```python
from build123d import *

# Parameters (mm, degrees)
BOSS_EXTRUDE1_DEPTH = 2
SKETCH2_R           = 10
CUT_EXTRUDE1_DEPTH  = 434.878349498
SKETCH4_OUTSIDE_W   = 492.732
SKETCH4_OUTSIDE_H   = 440.742
CUT_EXTRUDE2_DEPTH  = 3


with BuildPart() as part:
    # Sketch1 → Boss-Extrude1 (new body)
    with BuildSketch(Plane(origin=(0, 0, 0), x_dir=(1, 0, 0), z_dir=(0, 1, 0))):
        Polygon((-132.853430349, -388.070415552), (132.853430349, -388.070415552), (194.030344885, -282.108891325), (61.176914536, -52), (-61.176914536, -52), (-194.030344885, -282.108891325), align=None)
    extrude(amount=BOSS_EXTRUDE1_DEPTH)

    # Sketch2 → Cut-Extrude1 (cut, through all)
    with BuildSketch(Plane(origin=(0, 2, 0), x_dir=(1, 0, 0), z_dir=(0, 1, 0))):
        with Locations(Location((0, -240.726435625, 0), (0, 0, 270))):
            Circle(SKETCH2_R)
    extrude(amount=-CUT_EXTRUDE1_DEPTH, mode=Mode.SUBTRACT)

    # Sketch4 outside → Cut-Extrude2 (cut)
    with BuildSketch(Plane(origin=(0, 2, 0), x_dir=(1, 0, 0), z_dir=(0, 1, 0))):
        with Locations((0, -220.035)):
            Rectangle(SKETCH4_OUTSIDE_W, SKETCH4_OUTSIDE_H)
        Polygon((-75.405516164, -76.644660941), (-40.050177105, -112), (40.050177105, -112), (75.405516164, -76.644660941), (179.801743257, -257.464230384), (131.505451943, -270.405182639), (91.455274838, -339.774124237), (104.396227093, -388.070415552), (-104.396227093, -388.070415552), (-91.455274838, -339.774124237), (-131.505451943, -270.405182639), (-179.801743257, -257.464230384), align=None, mode=Mode.SUBTRACT)
    extrude(amount=-CUT_EXTRUDE2_DEPTH, mode=Mode.SUBTRACT)


solid = part.part
```
Source: CAD feature listing. Evaluate the final solid. Frame: model axes, mm. A direction names the side the tool comes from. Round coordinates to 2 decimals unless told otherwise and drop trailing zeros. Loops run counter-clockwise (first coordinate to the right, second up) from the corner with the lowest first, then second, coordinate; pieces in that order, holes last. Notation, with made-up numbers: M 6,-10.75 L 17,-10.75 A18 ccw 17,-5.75 Z; hole C 62,52.25 d7. An arc over 180 degrees is marked long. Use a Markdown table: item, result. Add a question column.
1. Set-up query: faces 4 (the flat face through (-98.016, 1.014, 364.26)), 5 (the flat face through (-57.98, 1.01, 94.07)), 6 (the flat face through (111.761, 1.014, 304.604)). Return all of +Z, -Z, +X, -X, +Y, -Y with unobstructed straight access to the full face (end or side cutting, diameter ignored); none if empty.
2. Cut plane D-D, the plane x = 64. Output: boundary loops of the cut face in (y, z), and give its area (3 significant figures).
3. Cut plane A-A, the plane x = 0. Output: boundary loops of the cut face in (y, z).
4. Cut plane B-B, the plane y = 1.05. Output: boundary loops of the cut face in (x, z).
5. Ray query, line 1 along Z through (x, y) = (-74, 0.2); line 2 along X through (y, z) = (1.15, 91); line 3 along X through (y, z) = (0.8, 245.5). Return the intervals inside material, ascending. Write a range as [from, to].
6. Cut plane C-C, the plane z = 295.5. Output: boundary loops of the cut face in (x, y), and give its area (3 significant figures).
7. Pull-direction query (X, two-part tool) for faces 1 (the flat face through (-126.873, 0.986, 165.789)), 2 (the flat face through (128.334, 0.986, 168.32)), 3 (the cylindrical face through (-3.83, 1.014, 249.964)); classes: +X half, -X half, draft (parallel to the pull), parting line (faces both ways), or undercut.
8. Contact query for a flat-ended pin moving along its axis: pin 1 (3 mm diameter, centred on x = -95, z = 339, fed in from -Y). Output: stop coordinate, or through.
Solution:
| question | item | result |
|---|---|---|
| 1 | face 4 | -X, +Y, -Y |
| 1 | face 5 | -Z, +Y, -Y |
| 1 | face 6 | +X, +Y, -Y |
| 2 | outline | M 0,88.05 L 2,88.05 L 2,388.07 L 0,388.07 Z |
| 2 | area | 600 mm2 |
| 3 | outline | M 0,112 L 2,112 L 2,230.73 L 0,230.73 Z; M 0,250.73 L 2,250.73 L 2,388.07 L 0,388.07 Z |
| 4 | outline | M -179.8,257.46 L -75.41,76.64 L -40.05,112 L 40.05,112 L 75.41,76.64 L 179.8,257.46 L 131.51,270.41 L 91.46,339.77 L 104.4,388.07 L -104.4,388.07 L -91.46,339.77 L -131.51,270.41 Z; hole C 0,240.73 d20 |
| 5 | line 1 | z = [78.05, 388.07] |
| 5 | line 2 | x = [-83.69, -61.05], [61.05, 83.69] |
| 5 | line 3 | x = [-172.89, -8.79], [8.79, 172.89] |
| 6 | outline | M -117.02,0 L 117.02,0 L 117.02,2 L -117.02,2 Z |
| 6 | area | 468 mm2 |
| 7 | face 1 | -X half |
| 7 | face 2 | +X half |
| 7 | face 3 | undercut |
| 8 | pin 1 | passes through |
